```python
from build123d import *

# Parameters (mm, degrees)
MAIN_BODY_DEPTH     = 172
SKETCH2_R           = 3.5
SKETCH3_R           = 2.5
SKETCH2_3_R         = 3.5
SKETCH3_3_R         = 2.5
SKETCH4_W           = 6
SKETCH4_H           = 76
SKETCH4_H_2         = 18
BOSS_EXTRUDE1_DEPTH = 16.5
CUT_EXTRUDE1_DEPTH  = 215.441717024
LPATTERN1_DEPTH     = 172


# Read off the part's stored shape, not the designer's step: Mirror2, LPattern1
with BuildPart() as part:
    # Sketch1 → Main Body (new body)
    with BuildSketch(Plane(origin=(0, 0, 0), x_dir=(1, 0, 0), z_dir=(0, 1, 0))):
        Polygon((-127, 0), (-127, 10), (-117, 10), (-117, 0.2), (-116, 0.2), (-116, 10), (116, 10), (116, 0.2), (117, 0.2), (117, 10), (127, 10), (127, 0), align=None)
    extrude(amount=MAIN_BODY_DEPTH)

    # Sketch2 → Cut-Loft2 section 0
    with BuildSketch(Plane(origin=(0, 0, -10), x_dir=(-1, 0, 0), z_dir=(0, 0, -1))):
        with Locations((103.5, 134)):
            Circle(SKETCH2_R)
    # Sketch3 → Cut-Loft2 section 1
    with BuildSketch(Plane.XY.offset(-5)):
        with Locations((-103.5, 134)):
            Circle(SKETCH3_R)
    cut_loft2 = loft(mode=Mode.SUBTRACT)

    # Sketch2<3> → Cut-Loft3 section 0
    with BuildSketch(Plane(origin=(0, 0, -10), x_dir=(-1, 0, 0), z_dir=(0, 0, -1))):
        with Locations((103.5, 38)):
            Circle(SKETCH2_3_R)
    # Sketch3<3> → Cut-Loft3 section 1
    with BuildSketch(Plane.XY.offset(-5)):
        with Locations((-103.5, 38)):
            Circle(SKETCH3_3_R)
    cut_loft3 = loft(mode=Mode.SUBTRACT)

    # Mirror1: Cut-Loft2, Cut-Loft3 across plane
    add(cut_loft2.mirror(Plane.XY.offset(-5)), mode=Mode.SUBTRACT)
    add(cut_loft3.mirror(Plane.XY.offset(-5)), mode=Mode.SUBTRACT)

    # Mirror2 outline → Mirror2 (revolve, cut)
    with BuildSketch(Plane(origin=(103.5, 134, 0), x_dir=(1, 0, 0), z_dir=(0, -1, 0))):
        Polygon((3.5, -10), (2.5, -5), (3.5, 0), (0, 0), (0, -10), align=None)
    revolve(axis=Axis((103.5, 134, 0), (0, 0, 1)), mode=Mode.SUBTRACT)

    # Mirror2 2 outline → Mirror2 2 (revolve, cut)
    with BuildSketch(Plane(origin=(103.5, 38, 0), x_dir=(1, 0, 0), z_dir=(0, -1, 0))):
        Polygon((3.5, -10), (2.5, -5), (3.5, 0), (0, 0), (0, -10), align=None)
    revolve(axis=Axis((103.5, 38, 0), (0, 0, 1)), mode=Mode.SUBTRACT)

    # Sketch4 → Boss-Extrude1 (add)
    with BuildSketch(Plane.XY):
        with Locations((100.5, 86)):
            Rectangle(SKETCH4_W, SKETCH4_H)
        with Locations((100.5, 153)):
            Rectangle(SKETCH4_W, SKETCH4_H_2)
        with Locations((100.5, 19)):
            Rectangle(SKETCH4_W, SKETCH4_H_2)
    boss_extrude1 = extrude(amount=BOSS_EXTRUDE1_DEPTH)

    # Mirror3: Boss-Extrude1 across plane
    add(boss_extrude1.mirror(Plane(origin=(0, 0, 0), x_dir=(0, 0, 1), z_dir=(1, 0, 0))))

    # Sketch5 → Cut-Extrude1 (cut, through all)
    with BuildSketch(Plane(origin=(0, 172, 0), x_dir=(1, 0, 0), z_dir=(0, 1, 0))):
        Polygon((129.5, 10.5), (127, 6.169872981), (124.5, 10.5), align=None)
    cut_extrude1 = extrude(amount=-CUT_EXTRUDE1_DEPTH, mode=Mode.SUBTRACT)

    # LPattern1 outline → LPattern1 (cut)
    with BuildSketch(Plane(origin=(0, 0, 0), x_dir=(1, 0, 0), z_dir=(0, 1, 0))):
        Polygon((119.788675135, 10), (122, 6.169872981), (124.211324865, 10), align=None)
        Polygon((117, 6.169872981), (119.211324865, 10), (117, 10), align=None)
        Polygon((116, 10), (114.788675135, 10), (116, 7.901923789), align=None)
    lpattern1 = extrude(amount=LPATTERN1_DEPTH, mode=Mode.SUBTRACT)

    # Mirror4: Cut-Extrude1, LPattern1 across plane
    add(cut_extrude1.mirror(Plane(origin=(0, 0, 0), x_dir=(0, 0, 1), z_dir=(1, 0, 0))), mode=Mode.SUBTRACT)
    add(lpattern1.mirror(Plane(origin=(0, 0, 0), x_dir=(0, 0, 1), z_dir=(1, 0, 0))), mode=Mode.SUBTRACT)


solid = part.part
```
The model under review builds one solid part; all positions refer to its coordinate system, in mm. A direction names the side the tool comes from. Round coordinates to 2 decimals unless told otherwise and drop trailing zeros. Write each loop counter-clockwise with the first axis right and the second up, starting at its lowest first coordinate (ties: lowest second). Pieces come first, ordered by that corner, then holes. Notation, with made-up numbers: (-24, -3.75) -> (35, -3.75) arc R13 cw to (35, 17.25) -> close; hole circle Ø4 at (59.5, 51). An arc over 180 degrees is marked (long way). Use CSV: the item, a comma, the result in double quotes.
Q1. For pin 1 Ø1.5 at (x, y) = (-74, 110) entering from +Z; pin 2 Ø5 at (x, z) = (-100.5, 8) entering from -Y; pin 3 Ø1.1 at (x, y) = (116.5, 115.5) entering from -Z; pin 4 Ø13 at (y, z) = (22.5, 6) entering from -X, all flat-tipped, find the tip position at first contact; note any pin that passes through.
Checks:
pin 1,"z = 0"
pin 2,"y = 10"
pin 3,"z = -7.99"
pin 4,"x = -127"
Q2. Consider section A-A (z = 4.25). Give the boundary of the cut face in (x, y), then the cut area to 3 significant figures.
Checks:
outline,"(-103.5, 10) -> (-97.5, 10) -> (-97.5, 28) -> (-103.5, 28) -> close; (-103.5, 48) -> (-97.5, 48) -> (-97.5, 124) -> (-103.5, 124) -> close; (-103.5, 144) -> (-97.5, 144) -> (-97.5, 162) -> (-103.5, 162) -> close; (97.5, 10) -> (103.5, 10) -> (103.5, 28) -> (97.5, 28) -> close; (97.5, 48) -> (103.5, 48) -> (103.5, 124) -> (97.5, 124) -> close; (97.5, 144) -> (103.5, 144) -> (103.5, 162) -> (97.5, 162) -> close"
area,"1,340 mm²"
Q3. Consider section C-C (y = 38). State how many separate pieces and enclosed holes the cut face has, then the cut area to 3 significant figures.
Checks:
separate pieces,"3"
enclosed holes,"0"
area,"2,360 mm²"
Q4. To check wall thickness, follow probe 1 along X at (y, z) = (10.5, -5); probe 2 along X at (y, z) = (49, -8.25); probe 3 along X at (y, z) = (118.5, 7.5). State the ranges of each line that lie inside material, in increasing order. Write a range as [from, to].
Checks:
probe 1,"[-127, -117], [-116, 116], [117, 127]"
probe 2,"[-125.8, -123.2], [-120.8, -118.2], [-115.8, 115.8], [118.2, 120.8], [123.2, 125.8]"
probe 3,"[-103.5, -97.5], [97.5, 103.5]"
Q5. Mouldability with a two-part tool opening along Y and no side actions: class faces 5 (the flat face through (116, 85, -4)), 6 (the flat face through (2, 172, -5)), 7 (the flat face through (-100, 28, 8)), 8 (the conical face through (-101.38, 39.95, -3.09)) as released by +Y, released by -Y, zero draft, split by the parting line, or undercut.
Checks:
face 5,"zero draft"
face 6,"released by +Y"
face 7,"undercut"
face 8,"undercut"
Q6. Consider section D-D (x = -9). Give the boundary of the cut face in (y, z).
Checks:
outline,"(0, -10) -> (172, -10) -> (172, 0) -> (0, 0) -> close"
Q7. For faces 1 (the flat face through (97.5, 153, 8)), 2 (the flat face through (-100, 10, 8)), 3 (the flat face through (-103.5, 153, 8)), 4 (the flat face through (100, 124, 8)), list the 3-axis set-ups (+Z, -Z, +X, -X, +Y, -Y) from which the entire face can be reached by the end or side of a thin tool; tool diameter is ignored.
Checks:
face 1,"+Z, +Y, -Y"
face 2,"+Z, +X, -X, -Y"
face 3,"+Z, -X, +Y, -Y"
face 4,"+Z, +X, -X"
